Study the drawing (mm; zero at the part's minimum x, y, z) and answer. Give positions to 0.01 mm unless a question says otherwise; leave off trailing zeros. Write each loop counter-clockwise with the first axis right and the second up, starting at its lowest first coordinate (ties: lowest second). Pieces come first, ordered by that corner, then holes. Notation, with made-up numbers: (48, 17) - (55, 17) arc R15 cw to (55, 26) - close; hole circle Ø9 at (36, 26.5). An arc over 180 degrees is marked (long way). Answer as CSV lines item,"result".
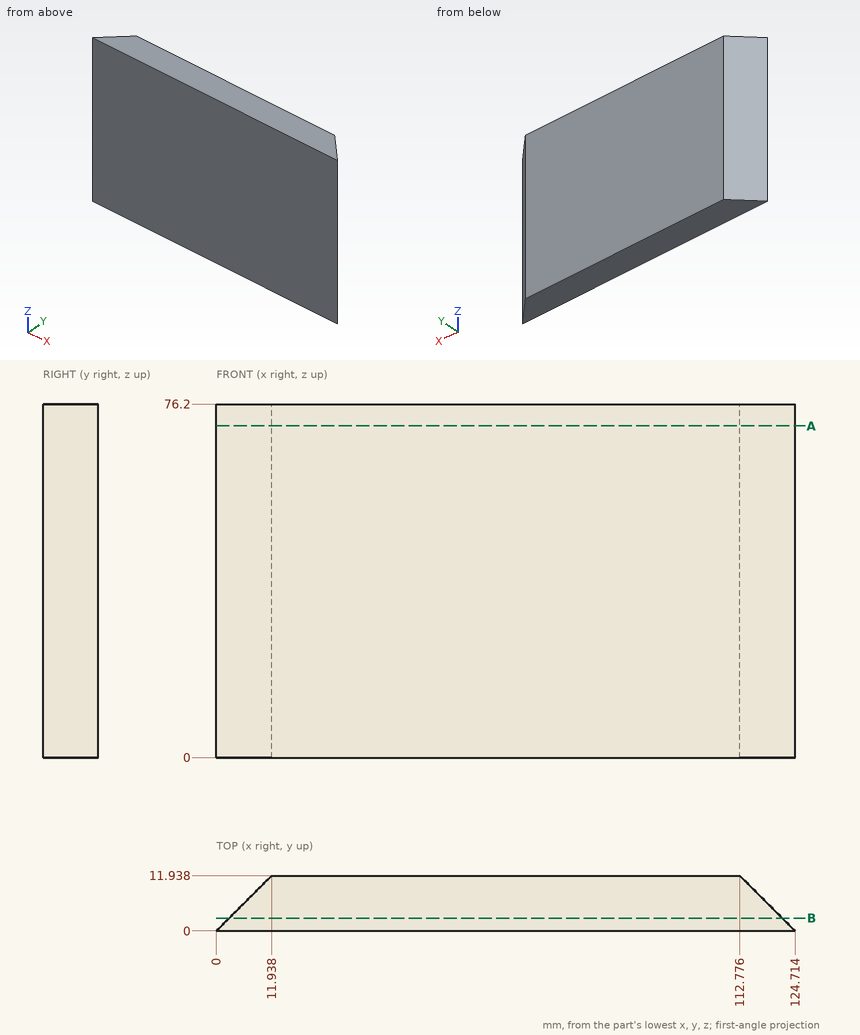
(1) A cutting plane is placed at B-B (y = 2.75). Write down the section's boundary in (x, z), and give its area (3 significant figures).
Worked out:
outline,"(2.75, 0) - (121.96, 0) - (121.96, 76.2) - (2.75, 76.2) - close"
area,"9,080 mm^2"
(2) Each of these flat-tipped pins is pushed along its axis until it touches: P1, Ø1, axis at y = 10.5, z = 63, coming from the -X side; P2, Ø1.5, axis at y = 4.5, z = 68, coming from the +X side. Where does it stop, or does it pass through?
Worked out:
P1,"stops at x = 10"
P2,"stops at x = 120.96"
(3) A cutting plane is placed at A-A (z = 71.5). Write down the section's boundary in (x, y), and give its area (3 significant figures).
Worked out:
outline,"(0, 0) - (124.71, 0) - (112.78, 11.94) - (11.94, 11.94) - close"
area,"1,350 mm^2"
(4) Find the intervals of material crossed by L1, parallel to X at y = 6, z = 19; L2, parallel to X at y = 3.75, z = 61, in increasing order.
Worked out:
L1,"x = 6 to 118.71"
L2,"x = 3.75 to 120.96"
